```python
from build123d import *

# Parameters (mm, degrees)
SKETCH1_R           = 1.6
BOSS_EXTRUDE1_DEPTH = 3
BOSS_EXTRUDE2_DEPTH = 3
FILLET1_R           = 0.5
CUT_EXTRUDE1_REACH  = 8
CHAMFER1_SIZE       = 3.5


with BuildPart() as part:
    # Sketch1 → Boss-Extrude1 (new body, symmetric)
    with BuildSketch(Plane.XY):
        Polygon((0, 0), (-21.213203436, 0), (0, 21.213203436), align=None)
        with Locations((-6.2, 6.2)):
            Circle(SKETCH1_R, mode=Mode.SUBTRACT)
    extrude(amount=BOSS_EXTRUDE1_DEPTH, both=True)

    # Sketch2 → Boss-Extrude2 (add, symmetric)
    with BuildSketch(Plane.XY):
        with BuildLine():
            Line((-9, 0), (-9, -6))
            Line((-9, -6), (-14, -6))
            Line((-14, -6), (-8.803847577, -15))
            Line((-8.803847577, -15), (10, -15))
            ThreePointArc((10, -15), (13.535533906, -13.535533906), (15, -10))
            Line((15, -10), (15, 8.803847577))
            Line((15, 8.803847577), (6, 14))
            Line((6, 14), (6, 9))
            Line((6, 9), (0, 9))
            Line((0, 9), (0, 0))
            Line((0, 0), (-9, 0))
        make_face()
    extrude(amount=BOSS_EXTRUDE2_DEPTH, both=True)

    # Fillet1
    fillet1_edges = [part.edges().sort_by_distance(p)[0] for p in [
        (-14, -6, 0),
        (-8.803847577, -15, 0),
        (15, 8.803847577, 0),
        (6, 14, 0),
    ]]
    fillet(fillet1_edges, radius=FILLET1_R)

    # Sketch4 → Cut-Extrude1 (cut, up to next)
    with BuildSketch(Plane.XY.offset(3), mode=Mode.PRIVATE) as cut_extrude1_sk1:
        Polygon((0, 9), (-6.106601718, 15.106601718), (0, 21.213203436), align=None)
    cut_extrude1_tool1 = extrude(cut_extrude1_sk1.sketch, amount=-CUT_EXTRUDE1_REACH, mode=Mode.PRIVATE) & part.part
    add(cut_extrude1_tool1.solids().sort_by_distance((-2.035534, 15.106602, 3))[0], mode=Mode.SUBTRACT)
    # Sketch4 → Cut-Extrude1 (cut, up to next)
    with BuildSketch(Plane.XY.offset(3), mode=Mode.PRIVATE) as cut_extrude1_sk2:
        Polygon((-21.213203436, 0), (-15.106601718, 6.106601718), (-9, 0), align=None)
    cut_extrude1_tool2 = extrude(cut_extrude1_sk2.sketch, amount=-CUT_EXTRUDE1_REACH, mode=Mode.PRIVATE) & part.part
    add(cut_extrude1_tool2.solids().sort_by_distance((-15.106602, 2.035534, 3))[0], mode=Mode.SUBTRACT)

    # Chamfer1
    chamfer1_edges = [part.edges().sort_by_distance(p)[0] for p in [
        (-6.106601718, 15.106601718, 0),
        (-15.106601718, 6.106601718, 0),
    ]]
    chamfer(chamfer1_edges, length=CHAMFER1_SIZE)


solid = part.part
```
Check sheet for the modelled part. Datum: model origin and axes. Units: mm. A direction names the side the tool comes from. Coordinates: 2 decimals unless noted, no trailing zeros. Loops run counter-clockwise (first coordinate to the right, second up) from the corner with the lowest first, then second, coordinate; pieces in that order, holes last.
1) Sectioned sample at B-B (z = -1.75). Record the boundary of the cut face in (x, y).
2) Sectioned sample at C-C (x = -6.2). Record the boundary of the cut face in (y, z), and give its area (3 significant figures).
3) Release check for a two-part mould opening along X. For faces 4 (the face through (1, -15, 0)), 5 (the face through (-2, 11, 0)), 6 (the face through (6, 11, 0)), 7 (the face through (-11.29, -10.69, 0.04)) record: released by +X, released by -X, zero draft, split by the parting line, or undercut.
4) Sectioned sample at D-D (x = 4.25). Record the boundary of the cut face in (y, z), and give its area (3 significant figures).
5) Gauge pin test, flat ends, axial feed: pin 1 (3 mm diameter, centred on x = -6.2, y = 6.2, fed in from -Z); pin 2 (2 mm diameter, centred on x = -12, z = 1.5, fed in from +Y); pin 3 (1.8 mm diameter, centred on x = 3.5, z = 0, fed in from +Y). Record the tip position at first contact, or that the pin passes through.
6) Material ranges on probe 1 along Y at (x, z) = (-6.2, -0.05); probe 2 along X at (y, z) = (-2.5, -2); probe 3 along Y at (x, z) = (3.75, 2), recorded low to high.
7) Sectioned sample at A-A (y = 6.2). Record the boundary of the cut face in (x, z).
8) Access from +Z, -Z, +X, -X, +Y, -Y to the whole of each face (thin tool, end or side, straight path). Record for faces 1 (the face through (3, 9, 0)), 2 (the face through (-11, 2, 0)), 3 (the face through (-6, 12.632, 0)).
Check sheet entries:
1. outline: (-13.57, -6.75) - (-8.95, -14.75) arc R0.5 ccw to (-8.52, -15) - (10, -15) arc R5 ccw to (15, -10) - (15, 8.52) arc R0.5 ccw to (14.75, 8.95) - (6.75, 13.57) arc R0.5 ccw to (6, 13.13) - (6, 9) - (0, 9) - (-3.63, 12.63) - (-8.58, 12.63) - (-12.63, 8.58) - (-12.63, 3.63) - (-9, 0) - (-9, -6) - (-13.13, -6) arc R0.5 ccw to start; hole circle Ø3.2 at (-6.2, 6.2)
2. outline: (-15, -3) - (4.6, -3) - (4.6, 3) - (-15, 3) - close; (7.8, -3) - (12.63, -3) - (12.63, 3) - (7.8, 3) - close
2. area: 147 mm2
3. face 4: zero draft
3. face 5: undercut
3. face 6: undercut
3. face 7: released by -X
4. outline: (-15, -3) - (9, -3) - (9, 3) - (-15, 3) - close
4. area: 144 mm2
5. pin 1: passes through
5. pin 2: stops at y = 10.21
5. pin 3: stops at y = 9
6. probe 1: y = -15 to 4.6, 7.8 to 12.63
6. probe 2: x = -9 to 15
6. probe 3: y = -15 to 9
7. outline: (-12.63, -3) - (-7.8, -3) - (-7.8, 3) - (-12.63, 3) - close; (-4.6, -3) - (15, -3) - (15, 3) - (-4.6, 3) - close
8. face 1: +Z, -Z, +Y
8. face 2: +Z, -Z, -X
8. face 3: +Z, -Z, -X, +Y
